Input: part model. Units: mm. Frame: model coordinates. Face numbers are marked on the shaded views. Coordinates: 2 decimals unless noted, no trailing zeros. Write each loop counter-clockwise with the first axis right and the second up, starting at its lowest first coordinate (ties: lowest second). Pieces come first, ordered by that corner, then holes.
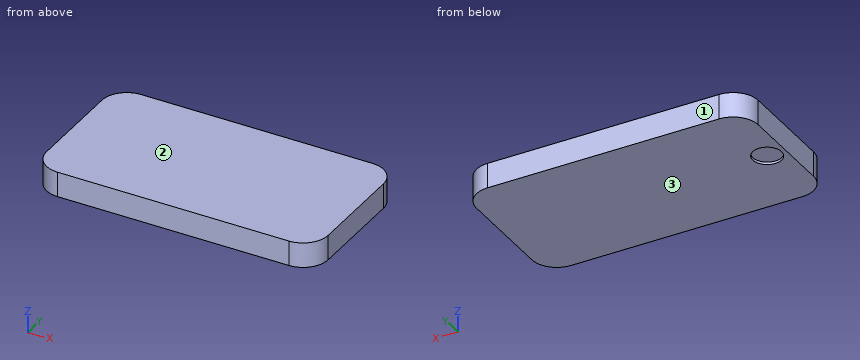
from build123d import *

# Parameters (mm, degrees)
F0_W     = 142.95493
F0_H     = 74.974402
F1_DEPTH = 12.7
F2_R     = 12.7
F3_R     = 7.313249
F4_DEPTH = 1.27


with BuildPart() as f1:
    # F0 (on Top) → F1 (new body)
    with BuildSketch(Plane.XY):
        Rectangle(F0_W, F0_H)
    extrude(amount=F1_DEPTH)

    # F2
    f2_edges = [f1.edges().sort_by_distance(p)[0] for p in [
        (71.477465, -37.487201, 6.35),
        (71.477465, 37.487201, 6.35),
        (-71.477465, 37.487201, 6.35),
        (-71.477465, -37.487201, 6.35),
    ]]
    fillet(f2_edges, radius=F2_R)

    # F3 (on face) → F4 (cut)
    with BuildSketch(Plane(origin=(0, 0, 0), x_dir=(1, 0, 0), z_dir=(0, 0, -1))):
        with Locations((-62.073462, 0)):
            Circle(F3_R)
    extrude(amount=-F4_DEPTH, mode=Mode.SUBTRACT)


solid = f1.part
Item 1: Material intervals for line 1 (X direction, y = 0, z = 0.6); line 2 (X direction, y = 28.5, z = 12.25); line 3 (X direction, y = 25, z = 7.25), sorted ascending.
Item 2: Pull-direction query (Z, two-part tool) for the marked faces 1, 2 and 3; classes: released by +Z, released by -Z, zero draft, split by the parting line, or undercut.
Item 3: Pin query (flat end, axial travel): pin 1 Ø11.5 at (x, y) = (-59, -2.5) entering from -Z. Return the tip coordinate at first contact, or that it passes through.
Item 4: Section query A-A, the plane y = -31. Return loops of the section in (x, z).
The answers:
1. line 1: x = -71.48 to -69.39, -54.76 to 71.48
1. line 2: x = -70.92 to 70.92
1. line 3: x = -71.48 to 71.48
2. face 1: zero draft
2. face 2: released by +Z
2. face 3: released by -Z
3. pin 1: stops at z = 0
4. outline: (-69.85, 0) - (69.85, 0) - (69.85, 12.7) - (-69.85, 12.7) - close
